Can you work these out from the model? Positions are in its coordinate system, mm. A direction names the side the tool comes from. Round coordinates to 2 decimals unless told otherwise and drop trailing zeros. Order: outer loops, then holes, each group sorted by start corner. A loop starts at its lowest first (then second) coordinate and runs counter-clockwise, first axis right, second up. Notation, with made-up numbers: (-18, 62.25) -> (40, 62.25) arc R23 ccw to (40, 96.25) -> close; hole circle Ø11 at (73.5, 69). An arc over 180 degrees is marked (long way). One line per item, written item: value.
```python
from build123d import *

# Parameters (mm, degrees)
BOSS_EXTRUDE1_DEPTH = 22
SKETCH6_W           = 12
SKETCH6_H           = 12
SKETCH6_W_2         = 22
BOSS_EXTRUDE4_DEPTH = 6
BOSS_EXTRUDE5_DEPTH = 22
SKETCH9_R           = 2
CUT_EXTRUDE9_DEPTH  = 6
SKETCH10_R          = 1.5
CUT_EXTRUDE10_DEPTH = 36
CUT_EXTRUDE11_DEPTH = 20


with BuildPart() as part:
    # Sketch1 → Boss-Extrude1 (new body)
    with BuildSketch(Plane.XY):
        Polygon((-36.238637744, 24.241346543), (-9.742760301, -30.758653457), (27.744579766, 24.241346543), align=None)
    extrude(amount=BOSS_EXTRUDE1_DEPTH)

    # Sketch6 → Boss-Extrude4 (add)
    with BuildSketch(Plane(origin=(-19.934259386, -9.603194429, 0), x_dir=(0, 0, 1), z_dir=(-0.9009094793526655, -0.4340070391278342, 0))):
        with Locations((28, 31.567082762)):
            Rectangle(SKETCH6_W, SKETCH6_H)
        with Locations((11, -29.48233592)):
            Rectangle(SKETCH6_W_2, SKETCH6_H)
    extrude(amount=-BOSS_EXTRUDE4_DEPTH)


with BuildPart() as boss_extrude4_piece_1:
    # of the separate pieces the step leaves, piece 1, a body of its own (boss_extrude4_pieces)
    add(part.part.solids().sort_by_distance((-36.238637744, 24.241346543, 0))[0])



with BuildPart() as boss_extrude4_piece_2:
    # of the separate pieces the step leaves, piece 2, a body of its own (boss_extrude4_pieces)
    add(part.part.solids().sort_by_distance((-4.337303425, -28.154611222, 0))[0])


with BuildPart() as boss_extrude4_piece_1_1:
    add(boss_extrude4_piece_1.part)

    add(boss_extrude4_piece_2.part)  # Boss-Extrude5 merges Boss-Extrude4 piece 2
    # Sketch8 → Boss-Extrude5 (add)
    with BuildSketch(Plane(origin=(0, 0, 0), x_dir=(-1, 0, 0), z_dir=(0, 0, -1))):
        Polygon((9.742760301, -30.758653457), (4.337303425, -28.154611222), (7.661322683, -27.704847324), align=None)
    extrude(amount=-BOSS_EXTRUDE5_DEPTH)

    # Sketch9 → Cut-Extrude9 (cut)
    with BuildSketch(Plane(origin=(-14.52880251, -6.999152194, 0), x_dir=(0, 0, -1), z_dir=(0.9009094793526653, 0.43400703912783434, 0))):
        with Locations(Location((-28, 30.567082762, 0), (0, 0, 90))):
            Circle(SKETCH9_R)
        with Locations(Location((-11, -29.48233592, 0), (0, 0, 90))):
            Circle(SKETCH9_R)
    extrude(amount=-CUT_EXTRUDE9_DEPTH, mode=Mode.SUBTRACT)

    # Sketch10 → Cut-Extrude10 (cut)
    with BuildSketch(Plane(origin=(7.662336774, -5.222556806, 0), x_dir=(0, 0, -1), z_dir=(0.8263158609823067, -0.5632069760656995, 0))):
        with Locations(Location((-7, -9.343049988, 0), (0, 0, 90))):
            Circle(SKETCH10_R)
    extrude(amount=-CUT_EXTRUDE10_DEPTH, mode=Mode.SUBTRACT)

    # Sketch12 → Cut-Extrude11 (cut)
    with BuildSketch(Plane(origin=(0, 0, 22), x_dir=(-1, 0, 0), z_dir=(0, 0, -1))):
        Polygon((30.833180868, 26.845388778), (29.578701161, 24.241346543), (36.238637744, 24.241346543), align=None)
    extrude(amount=-CUT_EXTRUDE11_DEPTH, mode=Mode.SUBTRACT)


solid = boss_extrude4_piece_1_1.part
```
Q1. I want a section at C-C on y = 11.5. List the corners of the cut face in (x, z) for me.
Answers below:
outline: (-30.1, 0) -> (19.06, 0) -> (19.06, 22) -> (-30.1, 22) -> close
Q2. I want a section at B-B on x = 13.5. List the corners of the cut face in (y, z) for me.
Answers below:
outline: (3.34, 0) -> (24.24, 0) -> (24.24, 22) -> (3.34, 22) -> close
Q3. Please list where these lines run through material, in increasing order: line 1 along Z through (x, y) = (-1, 3); line 2 along Y through (x, z) = (-4.5, 12); line 3 along X through (y, z) = (-7.5, 7).
Answers below:
line 1: 0 to 22
line 2: -41.55 to -36.82, -32.97 to -28.13, -23.07 to 24.24
line 3: -20.95 to -8.25, -2.92 to 6.11
Q4. We'd pull the mould along X, two halves only. Please class faces 1 (the face through (-27.15, 7.62, 7.02)), 2 (the face through (-2, 6, 22)), 3 (the face through (-1.77, -33.48, 13.29)): released by +X, released by -X, zero draft, split by the parting line, or undercut.
Answers below:
face 1: undercut
face 2: zero draft
face 3: released by +X
Q5. Will these pins go through, and if not, where does the flat tip stop? pin 1 Ø5 at (y, z) = (4.5, 11.5) entering from +X; pin 2 Ø17.5 at (x, y) = (11.5, -2.5) entering from +Z; pin 3 Ø2 at (x, z) = (-18.5, 24) entering from -Y; pin 4 Ø1 at (y, z) = (-31.5, 10) entering from +X.
Answers below:
pin 1: x = 15.99
pin 2: z = 22
pin 3: through
pin 4: x = -2.48
Q6. On a 3-axis mill with a long thin cutter (end or side, diameter ignored), from which of +Z, -Z, +X, -X, +Y, -Y can I reach the whole of each face in a straight line? I mean faces 4 (the face through (-11.875, -2.375, 5.669)), 5 (the face through (-1.9, -40.3, 10.8)), 6 (the face through (-26.75, 18.37, 27.92)), 7 (the face through (9.79, -2.1, 10.85)), 8 (the face through (-28.37, 14.71, 27.92)). Say none if no direction works.
Answers below:
face 4: none
face 5: +Z, -Z, +X, -Y
face 6: +Z, +X, +Y
face 7: +Z, -Z, +X
face 8: +Z, +X, -Y
Q7. I want a section at A-A on z = 3.5. List the corners of the cut face in (x, y) for me, plus the area to 3 significant figures.
Answers below:
outline: (-36.24, 24.24) -> (-4.53, -41.57) -> (0.87, -38.97) -> (-4.34, -28.15) -> (-7.66, -27.7) -> (27.74, 24.24) -> close
area: 1,840 mm^2
